Here's how the part is built. I have some questions about the finished solid (model axes, mm). Give positions to 0.01 mm unless a question says otherwise; leave off trailing zeros. Write each loop counter-clockwise with the first axis right and the second up, starting at its lowest first coordinate (ties: lowest second). Pieces come first, ordered by that corner, then holes. Notation, with made-up numbers: (34, -20) -> (66, -20) arc R12 ccw to (66, -11) -> close; hole circle Ø4 at (-19.5, 73). An arc over 180 degrees is marked (long way). Use CSV: the item, a comma, the result in double quotes. Start each with the question number.
(1) I need wall thicknesses on L1, parallel to Y at x = -0.35, z = 0; L2, parallel to Y at x = 0.25, z = 0.1; L3, parallel to X at y = -1.75, z = -0.9. Which ranges of each line are inside material? Lowest first, please. Write a range as [from, to].
(2) For pin 1 Ø1 at (y, z) = (7, 1) entering from +X; pin 2 Ø1.5 at (y, z) = (-1, -1.5) entering from -X, each with a flat end and sliding along its axis, tell me the tip position at first contact or that it passes through.
(3) Suppose I cut it at D-D on z = 0.4. List the corners of the cut face in (x, y) for me.
(4) Suppose I cut it at B-B on x = -0.7. List the corners of the cut face in (y, z) for me.
(5) Suppose I cut it at A-A on z = 1.27. List the corners of the cut face in (x, y) for me (1 decimal), plus the area to 3 significant figures.
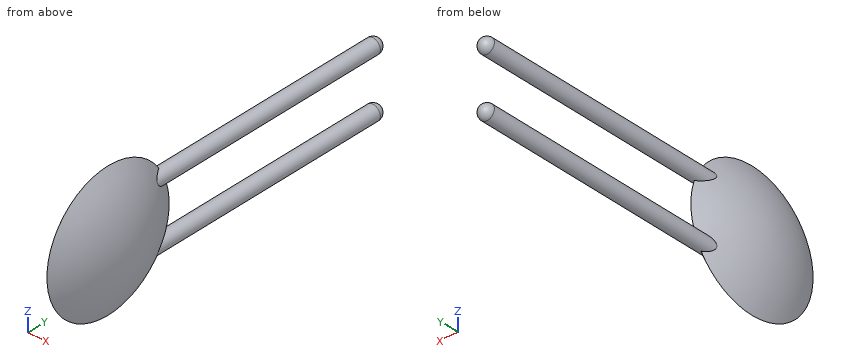
Autodesk Inventor part; units mm, degrees
ref_plane "YZ Plane" through (0, 0, 0) normal (1, 0, 0) x (0, 1, 0)
ref_plane "XZ Plane" through (0, 0, 0) normal (0, 1, 0) x (-1, 0, 0)
ref_plane "XY Plane" through (0, 0, 0) normal (0, 0, 1) x (1, 0, 0)
sketch "Náčrt3" plane through (0, 0, 0) normal (0, 1, 0) x (-1, 0, 0)
  arc A0 (0, -2.8575) -> (0.9525, 0) centre (-3.81, 0) ccw
  arc A1 (-0.9525, 0) -> (0, -2.8575) centre (3.81, 0) ccw
  line L0 (0.9525, 0) -> (-0.9525, 0)
  point P0 (0, 0)
revolve "Rotace1" add sketch "Náčrt3" angle 360 about axis through (-0.9525, 0, 0) along (1, 0, 0)
sketch "Náčrt4" plane through (0, 0, 0) normal (0, 1, 0) x (-1, 0, 0)
  circle A0 centre (0, -1.27) radius 0.3175
  circle A1 centre (0, 1.27) radius 0.3175
  point P0 (0, 0)
  dimension "d6" = 0.635
  dimension "d7" = 0.635
  dimension "d8" = 2.54
  dimension "d9" = 1.27
extrude "Vysunutí2" add sketch "Náčrt4" along normal blind 12.7
fillet "Zaoblení1" radius 0.3175 2 edges at (0.3175, 12.7, 1.27) (0.3175, 12.7, -1.27)
properties part number "Ceramic-Capacitor"
Geometry says:
1,L1,"[-2.32, 2.32]"
1,L2,"[-2.49, 2.49]"
1,L3,"[-0.53, 0.53]"
2,pin 1,"x = 0.32"
2,pin 2,"x = -0.83"
3,outline,"(0, -2.83) arc R4.75 ccw to (0, 2.83) arc R4.75 ccw to start"
4,outline,"circle Ø3.06 at (0, 0)"
5,outline,"(-0.3, 2) arc R4.6 ccw to (0, -2.6) arc R4.6 ccw to (0.3, 2) -> (0.3, 12.4) arc R0.3 ccw to (-0.3, 12.4) -> close"
5,area,"12.0 mm²"
